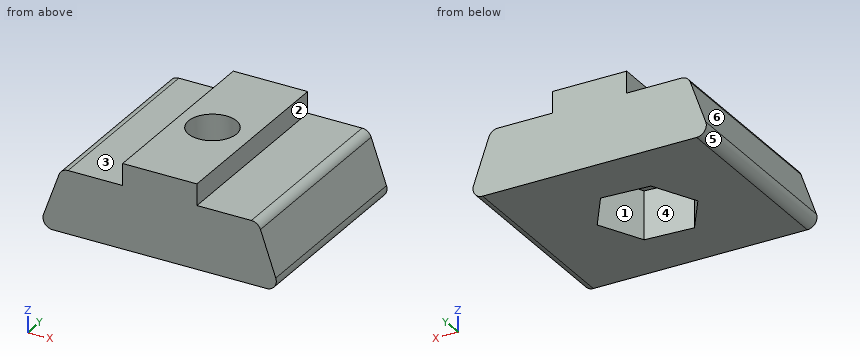
from build123d import *

# Parameters (mm, degrees)
F1_DEPTH = 25.4
F3_D     = 6.35
F4_R     = 3.175
F5_DEPTH = 6.35
F6_R     = 1.27


with BuildPart() as f1:
    # F0 (on Front) → F1 (new body)
    with BuildSketch(Plane.XZ):
        Polygon((-12.6819006406, 8.255), (-15.624309808, 0), (16.125690192, 0), (13.2260993594, 8.3013381809), (5.1634775414, 8.3013381809), (5.1634775414, 11.1125), (-4.6192788226, 11.1125), (-4.6192788226, 8.255), align=None)
    extrude(amount=F1_DEPTH)

    # F3 (through all)
    with Locations(Plane.XY.offset(11.1125)):
        with Locations((0, -12.8323249519)):
            Hole(F3_D / 2)

    # F4 (on face) → F5 (cut)
    with BuildSketch(Plane(origin=(0, 0, 0), x_dir=(1, 0, 0), z_dir=(0, 0, -1))):
        Polygon((-6.4124855846, 13.2020820447), (-3.5264618279, 7.4638280807), (2.8860237566, 7.0940709878), (6.4124855846, 12.462567859), (3.5264618279, 18.2008218231), (-2.8860237566, 18.570578916), align=None)
        with Locations((0, 12.8323249519)):
            Circle(F4_R, mode=Mode.SUBTRACT)
    extrude(amount=-F5_DEPTH, mode=Mode.SUBTRACT)

    # F6
    f6_edges = [f1.edges().sort_by_distance(p)[0] for p in [
        (16.12569, -12.7, 0),
        (-15.62431, -12.7, 0),
        (13.226099, -12.7, 8.301338),
        (-12.681901, -12.7, 8.255),
    ]]
    fillet(f6_edges, radius=F6_R)


solid = f1.part
Geometry: final body of the model. Coordinates: model frame, mm. Face numbers are marked on the shaded views. A direction names the side the tool comes from. Round coordinates to 2 decimals unless told otherwise and drop trailing zeros. Order: outer loops, then holes, each group sorted by start corner. A loop starts at its lowest first (then second) coordinate and runs counter-clockwise, first axis right, second up.
Q1. Section B-B, the plane y = -2.5. Output: boundary loops of the cut face in (x, z) (1 decimal).
Result sheet:
outline: (-15, 1.7) arc R1.3 ccw to (-13.8, 0) - (14.3, 0) arc R1.3 ccw to (15.5, 1.7) - (13.5, 7.5) arc R1.3 ccw to (12.3, 8.3) - (5.2, 8.3) - (5.2, 11.1) - (-4.6, 11.1) - (-4.6, 8.3) - (-11.8, 8.3) arc R1.3 ccw to (-13, 7.4) - close
Q2. Section C-C, the plane z = 3. Output: boundary loops of the cut face in (x, y) (3 decimals).
Result sheet:
outline: (-14.555, -25.4) - (15.078, -25.4) - (15.078, 0) - (-14.555, 0) - close; hole (-6.412, -13.202) - (-2.886, -18.571) - (3.526, -18.201) - (6.412, -12.463) - (2.886, -7.094) - (-3.526, -7.464) - close
Q3. Mould query, pull axis Z, two halves, no side actions, for the marked faces 4, 5 and 6. Classes: released by +Z, released by -Z, zero draft, split by the parting line, or undercut.
Result sheet:
face 4: zero draft
face 5: split by the parting line
face 6: released by +Z
Q4. Section A-A, the plane x = 0. Output: boundary loops of the cut face in (y, z).
Result sheet:
outline: (-25.4, 0) - (-18.4, 0) - (-18.4, 6.35) - (-16.01, 6.35) - (-16.01, 11.11) - (-25.4, 11.11) - close; (-9.66, 6.35) - (-7.26, 6.35) - (-7.26, 0) - (0, 0) - (0, 11.11) - (-9.66, 11.11) - close
Q5. Section D-D, the plane z = 5.25. Output: boundary loops of the cut face in (x, y).
Result sheet:
outline: (-13.75, -25.4) - (14.29, -25.4) - (14.29, 0) - (-13.75, 0) - close; hole (-6.41, -13.2) - (-2.89, -18.57) - (3.53, -18.2) - (6.41, -12.46) - (2.89, -7.09) - (-3.53, -7.46) - close
Q6. Access query for the marked faces 1, 2 and 3. Directions: +Z, -Z, +X, -X, +Y, -Y. A direction counts if a zero-diameter tool reaches every point of the face in a straight line with its end or side. Return the directions, or none.
Result sheet:
face 1: -Z
face 2: +Z, +X, +Y, -Y
face 3: +Z, -X, +Y, -Y
Q7. Pin query (flat end, axial travel): pin 1 (3 mm diameter, centred on y = -9.5, z = 9.5, fed in from -X); pin 2 (0.9 mm diameter, centred on y = -10.5, z = 10, fed in from -X); pin 3 (2 mm diameter, centred on x = -7, y = -13, fed in from +Z) (3 decimals); pin 4 (5 mm diameter, centred on x = 0, y = -12.83, fed in from -Z). Return the tip coordinate at first contact, or that it passes through.
Result sheet:
pin 1: stops at x = -12.55
pin 2: stops at x = -4.62
pin 3: stops at z = 8.255
pin 4: passes through
Q8. Material intervals for probe 1 along Y at (x, z) = (0, 8.3); probe 2 along Z at (x, y) = (-9.5, -15.75) (3 decimals); probe 3 along X at (y, z) = (-12, 10.5), sorted ascending.
Result sheet:
probe 1: y = -25.4 to -16.01, -9.66 to 0
probe 2: z = 0 to 8.255
probe 3: x = -4.62 to -3.06, 3.06 to 5.16
